from build123d import *

# Parameters (mm, degrees)
F0_W      = 102.6049330831
F0_H      = 60.307007283
F1_DEPTH  = 42.672
F2_W      = 50.8497301489
F2_H      = 23.2719845266
F3_DEPTH  = 108.712
F4_W      = 21.308818832
F4_H      = 44.3562362343
F5_DEPTH  = 70.612
F6_W      = 50.8497301489
F6_H      = 44.3562362343
F7_DEPTH  = 37.592
F8_W      = 21.4821361005
F8_H      = 44.3062051199
F9_DEPTH  = 71.882
F10_R     = 5.5376210479
F11_DEPTH = 182.626


with BuildPart() as f1:
    # F0 (on Top) → F1 (new body)
    with BuildSketch(Plane.XY):
        with Locations((-2.9272511601, -17.3868890852)):
            Rectangle(F0_W, F0_H)
    extrude(amount=F1_DEPTH)

    # F2 (on face) → F3 (cut)
    with BuildSketch(Plane.XZ.offset(47.5403927267)):
        with Locations((-3.8559036329, 31.0360077367)):
            Rectangle(F2_W, F2_H)
    extrude(amount=-F3_DEPTH, mode=Mode.SUBTRACT)

    # F4 (on face) → F5 (cut)
    with BuildSketch(Plane.XY.offset(42.672)):
        with Locations((-39.9351781234, -15.4247684404)):
            Rectangle(F4_W, F4_H)
    extrude(amount=-F5_DEPTH, mode=Mode.SUBTRACT)

    # F6 (on face) → F7 (cut)
    with BuildSketch(Plane.XY.offset(19.4000154734)):
        with Locations((-3.8559036329, -15.4247684404)):
            Rectangle(F6_W, F6_H)
    extrude(amount=-F7_DEPTH, mode=Mode.SUBTRACT)

    # F8 (on face) → F9 (cut)
    with BuildSketch(Plane.XY.offset(42.672)):
        with Locations((32.3100294918, -15.2362354565)):
            Rectangle(F8_W, F8_H)
    extrude(amount=-F9_DEPTH, mode=Mode.SUBTRACT)

    # F10 (on face) → F11 (cut)
    with BuildSketch(Plane.YZ.offset(48.3752153814)):
        with Locations((-17.9856810719, 23.4969127923)):
            Circle(F10_R)
    extrude(amount=-F11_DEPTH, mode=Mode.SUBTRACT)


solid = f1.part
Work out the finished part from the listing and answer in its coordinate system (mm). A direction names the side the tool comes from. Coordinates: 2 decimals unless noted, no trailing zeros. Loops run counter-clockwise (first coordinate to the right, second up) from the corner with the lowest first, then second, coordinate; pieces in that order, holes last. Notation, with made-up numbers: (-2.5, 47) -> (48.5, 47) arc R16 cw to (48.5, 51) -> close; hole circle Ø8 at (31, 58.5). An arc over 180 degrees is marked (long way). Write each question's results on one line, items separated by ' | '. Start each with the question number.
1) Find section C-C on z = 34.5. Determine the outline of the cut face in (x, y), then the cut area to 3 significant figures.
2) Find section A-A on y = -0.5. Determine the outline of the cut face in (x, z), then the cut area to 3 significant figures.
3) Consider line 1 along Y through (x, z) = (15.5, 15); line 2 along Y through (x, z) = (29.5, 4.5); line 3 along X through (y, z) = (-29, 33). Determine where each line is inside the solid, lowest interval first.
4) Find section B-B on x = 25. Determine the outline of the cut face in (y, z), then the cut area to 3 significant figures.
5) The mould has two halves that part along Y. Classify faces 4 (the cylindrical face through (-52.384, -18.707, 28.987)), 5 (the flat face through (21.569, 10, 31)), 6 (the flat face through (-4, -47.54, 16)): pulls with the +Y half, pulls with the -Y half, needs draft (parallel to the pull), parting line crosses it, or undercut.
6) Find section D-D on z = 20.5. Determine the outline of the cut face in (x, y).
7) Flat-ended cylindrical pins translate along their axes: P1, Ø5, axis at x = -14, y = 9.5, coming from the +Z side; P2, Ø12.5, axis at y = -17.99, z = 23.5, coming from the +X side. Find the tip coordinate at first contact, or state that the pin passes through.
8) For faces 1 (the flat face through (-54.23, -18, 16)), 2 (the flat face through (-4, -43, 19.4)), 3 (the flat face through (-23, -37.603, 17)), determine the directions among +Z, -Z, +X, -X, +Y, -Y from which every point of the face is accessible in a straight line to the end or side of a thin tool.
Response values:
1) outline: (-54.23, -47.54) -> (-29.28, -47.54) -> (-29.28, -37.6) -> (-50.59, -37.6) -> (-50.59, 6.75) -> (-29.28, 6.75) -> (-29.28, 12.77) -> (-54.23, 12.77) -> close; (21.57, -47.54) -> (48.38, -47.54) -> (48.38, 12.77) -> (21.57, 12.77) -> (21.57, 6.92) -> (43.05, 6.92) -> (43.05, -37.39) -> (21.57, -37.39) -> close | area: 1,220 mm^2
2) outline: (-54.23, 0) -> (-50.59, 0) -> (-50.59, 42.67) -> (-54.23, 42.67) -> close; (43.05, 0) -> (48.38, 0) -> (48.38, 42.67) -> (43.05, 42.67) -> close | area: 383 mm^2
3) line 1: y = -47.54 to -37.6, 6.75 to 12.77 | line 2: y = -47.54 to -37.39, 6.92 to 12.77 | line 3: x = -54.23 to -50.59, 43.05 to 48.38
4) outline: (-47.54, 0) -> (-37.39, 0) -> (-37.39, 42.67) -> (-47.54, 42.67) -> close; (6.92, 0) -> (12.77, 0) -> (12.77, 42.67) -> (6.92, 42.67) -> close | area: 683 mm^2
5) face 4: undercut | face 5: needs draft | face 6: pulls with the -Y half
6) outline: (-54.23, -47.54) -> (-29.28, -47.54) -> (-29.28, -37.6) -> (-50.59, -37.6) -> (-50.59, -22.64) -> (-54.23, -22.64) -> close; (-54.23, -13.33) -> (-50.59, -13.33) -> (-50.59, 6.75) -> (-29.28, 6.75) -> (-29.28, 12.77) -> (-54.23, 12.77) -> close; (21.57, -47.54) -> (48.38, -47.54) -> (48.38, -22.64) -> (43.05, -22.64) -> (43.05, -37.39) -> (21.57, -37.39) -> close; (21.57, 6.92) -> (43.05, 6.92) -> (43.05, -13.33) -> (48.38, -13.33) -> (48.38, 12.77) -> (21.57, 12.77) -> close
7) P1: stops at z = 19.4 | P2: stops at x = 48.38
8) face 1: +Z, -Z, -X, +Y, -Y | face 2: +Z, +Y, -Y | face 3: +Z, -Z
